Design review of the part built by this model. Coordinates are the model's own, in mm. A direction names the side the tool comes from. Round coordinates to 2 decimals unless told otherwise and drop trailing zeros. Write each loop counter-clockwise with the first axis right and the second up, starting at its lowest first coordinate (ties: lowest second). Pieces come first, ordered by that corner, then holes. Notation, with made-up numbers: (-11.5, 47.5) -> (39.5, 47.5) arc R22 ccw to (39.5, 78.5) -> close; hole circle Ø6 at (-28, -6.75). An arc over 180 degrees is marked (long way). Write item = value, one per line. Start each with the question number.
Item 1: For pin 1 Ø6 at (x, y) = (2.5, -38.5) entering from -Z; pin 2 Ø4 at (x, z) = (1, 1) entering from +Y; pin 3 Ø2 at (y, z) = (8, -8) entering from -X, all flat-tipped, find the tip position at first contact; note any pin that passes through.
Item 2: Add section C-C, the plane y = 52. State the section outline as (x, z) points.
Item 3: Machinability: for faces 1 (the cylindrical face through (-6, 30, 0)), 2 (the flat face through (0, 48.5, 0)), 3 (the flat face through (-5, 0, 2)), 4 (the flat face through (5, 60.5, 10)), 5 (the cylindrical face through (-11.99, 39.93, -0.53)), which of the approach directions +Z, -Z, +X, -X, +Y, -Y give a long, thin tool a straight path to every point of the face, cutting with its end or side? Answer none if there is none.
Item 4: Mouldability with a two-part tool opening along Y and no side actions: class faces 6 (the cylindrical face through (-2.17, 12.32, 9.76)), 7 (the flat face through (0, -50, 0)), 8 (the flat face through (6, 45, 10)) as released by +Y, released by -Y, zero draft, split by the parting line, or undercut.
Item 5: Add section A-A, the plane x = 0. State the section outline as (y, z) points, then the cut area to 3 significant figures.
Item 6: To check wall thickness, follow L1, parallel to Y at x = -1.25, z = -8; L2, parallel to X at y = 53.5, z = 0; L3, parallel to Y at x = -7, z = -9.25. State the ranges of each line that lie inside material, in increasing order.
Item 7: Add section B-B, the plane z = 0. State the section outline as (x, y) points.
Item 8: Add section D-D, the plane x = -8.75. State the section outline as (y, z) points.
from build123d import *

# Parameters (mm, degrees)
SKETCH_1_R          = 10
EXTRUDE_1_DEPTH     = 25
SKETCH_2_R          = 5
EXTRUDE_2_DEPTH     = 50
SKETCH_3_R          = 6
EXTRUDE_3_DEPTH     = 10
SKETCH_4_R          = 12
EXTRUDE_4_DEPTH     = 10
EXTRUDE_START       = 0.5
SKETCH_5_R          = 12
EXTRUDE_5_DEPTH     = 15
SKETCH_6_R          = 11.5
EXTRUDE_6_DEPTH     = 1
SKETCH_7_R          = 11
CUT_EXTRUDE_1_DEPTH = 12


with BuildPart() as part:
    # Sketch 1 → Extrude 1 (new body)
    with BuildSketch(Plane(origin=(0, 0, 0), x_dir=(1, 0, 0), z_dir=(0, 1, 0))):
        Circle(SKETCH_1_R)
    extrude(amount=EXTRUDE_1_DEPTH)

    # Sketch 2 → Extrude 2 (add)
    with BuildSketch(Plane.XZ):
        Circle(SKETCH_2_R)
    extrude(amount=EXTRUDE_2_DEPTH)

    # Sketch 3 → Extrude 3 (add)
    with BuildSketch(Plane(origin=(0, 25, 0), x_dir=(1, 0, 0), z_dir=(0, 1, 0))):
        Circle(SKETCH_3_R)
    extrude(amount=EXTRUDE_3_DEPTH)

    # Sketch 4 → Extrude 4 (add)
    with BuildSketch(Plane(origin=(0, 35, 0), x_dir=(1, 0, 0), z_dir=(0, 1, 0))):
        Circle(SKETCH_4_R)
    extrude(amount=EXTRUDE_4_DEPTH)



with BuildPart() as body_2:
    # Sketch 5 → Extrude 5 (new body)
    with BuildSketch(Plane(origin=(0, 45, 0), x_dir=(1, 0, 0), z_dir=(0, 1, 0)).offset(EXTRUDE_START)):
        Circle(SKETCH_5_R)
    extrude(amount=EXTRUDE_5_DEPTH)


with BuildPart() as part_1:
    add(part.part)

    add(body_2.part)  # Extrude 6 merges body 2
    # Sketch 6 → Extrude 6 (add)
    with BuildSketch(Plane(origin=(0, 45, 0), x_dir=(1, 0, 0), z_dir=(0, 1, 0))):
        Circle(SKETCH_6_R)
    extrude(amount=EXTRUDE_6_DEPTH)

    # Sketch 7 → Cut-Extrude 1 (cut)
    with BuildSketch(Plane(origin=(0, 60.5, 0), x_dir=(1, 0, 0), z_dir=(0, 1, 0))):
        Circle(SKETCH_7_R)
    extrude(amount=-CUT_EXTRUDE_1_DEPTH, mode=Mode.SUBTRACT)


solid = part_1.part
Result set:
q1.pin_1 = -5
q1.pin_2 = 48.5
q1.pin_3 = -7.14
q2.outline = circle Ø24 at (0, 0); hole circle Ø22 at (0, 0)
q3.face_1 = none
q3.face_2 = +Y
q3.face_3 = -Y
q3.face_4 = +Z, -Z, +X, -X, +Y
q3.face_5 = +Y, -Y
q4.face_6 = zero draft
q4.face_7 = released by -Y
q4.face_8 = undercut
q5.outline = (-50, -5) -> (0, -5) -> (0, -10) -> (25, -10) -> (25, -6) -> (35, -6) -> (35, -12) -> (45, -12) -> (45, -11.5) -> (45.5, -11.5) -> (45.5, -12) -> (60.5, -12) -> (60.5, -11) -> (48.5, -11) -> (48.5, 11) -> (60.5, 11) -> (60.5, 12) -> (45.5, 12) -> (45.5, 11.5) -> (45, 11.5) -> (45, 12) -> (35, 12) -> (35, 6) -> (25, 6) -> (25, 10) -> (0, 10) -> (0, 5) -> (-50, 5) -> close
q5.area = 1,470 mm²
q6.L1 = 0 to 25, 35 to 48.5
q6.L2 = -12 to -11, 11 to 12
q6.L3 = 35 to 45, 45.5 to 60.5
q7.outline = (-12, 35) -> (-6, 35) -> (-6, 25) -> (-10, 25) -> (-10, 0) -> (-5, 0) -> (-5, -50) -> (5, -50) -> (5, 0) -> (10, 0) -> (10, 25) -> (6, 25) -> (6, 35) -> (12, 35) -> (12, 45) -> (11.5, 45) -> (11.5, 45.5) -> (12, 45.5) -> (12, 60.5) -> (11, 60.5) -> (11, 48.5) -> (-11, 48.5) -> (-11, 60.5) -> (-12, 60.5) -> (-12, 45.5) -> (-11.5, 45.5) -> (-11.5, 45) -> (-12, 45) -> close
q8.outline = (0, -4.84) -> (25, -4.84) -> (25, 4.84) -> (0, 4.84) -> close; (35, -8.21) -> (45, -8.21) -> (45, -7.46) -> (45.5, -7.46) -> (45.5, -8.21) -> (60.5, -8.21) -> (60.5, -6.67) -> (48.5, -6.67) -> (48.5, 6.67) -> (60.5, 6.67) -> (60.5, 8.21) -> (45.5, 8.21) -> (45.5, 7.46) -> (45, 7.46) -> (45, 8.21) -> (35, 8.21) -> close
